CAD build for the part. Positions are in the model's coordinates, mm. A direction names the side the tool comes from. Give positions to 0.01 mm unless a question says otherwise; leave off trailing zeros. Write each loop counter-clockwise with the first axis right and the second up, starting at its lowest first coordinate (ties: lowest second). Pieces come first, ordered by that corner, then holes. Notation, with made-up numbers: (27, 76) - (72, 76) arc R19 ccw to (72, 94) - close; hole circle Ø9 at (-7, 42.25). An arc over 180 degrees is marked (long way). Put each result on its own line as item: value. Start each with the question number.
1. Cut at B-B on x = 0. List the corners of the cut face in (y, z).
2. Mould opens along Y. For faces 1 (the cylindrical face through (-3.88, -17.48, -12.64)), 2 (the flat face through (-4.89, 14, -19)), 3 (the flat face through (-8, -15, -5.426)) say: +Y half, -Y half, draft (parallel to the pull), parting line (faces both ways), or undercut.
3. Drop flat-ended pins along their axis: pin 1 (3 mm diameter, centred on y = 8, z = -9, fed in from +X); pin 2 (8 mm diameter, centred on x = 13.5, z = -18, fed in from -Y); pin 3 (16 mm diameter, centred on x = -5, y = -5.5, fed in from +Z). Give the stop position or say it passes through.
4. Cut at C-C on y = 9.5. List the corners of the cut face in (x, z).
5. Cut at A-A on y = 0. List the corners of the cut face in (x, z), and give its area (3 significant figures).
6. Tool access for faces 4 (the flat face through (4.9, -12.2, -18.126)), 5 (the flat face through (4.89, 14, -19)), 6 (the flat face through (-1.4, -13.2, -19.65)): list every direction of +Z, -Z, +X, -X, +Y, -Y with a clear straight run to the whole face (end or side of a thin tool).
7. Cut at D-D on z = -9.5. List the corners of the cut face in (x, y), and give its area (3 significant figures).
8. Wall check: line 1 (Y direction, x = 0, z = -10.75); line 2 (Z direction, x = -10, y = 12.5); line 3 (X direction, y = -12.5, z = -14). Give the ranges that are in metal, low to high.
from build123d import *

# Parameters (mm, degrees)
CUT_EXTRUDE1_DEPTH = 15.224


with BuildPart() as part:
    # Sketch1 → Revolve1 (revolve)
    with BuildSketch(Plane(origin=(0, 0, 0), x_dir=(1, 0, 0), z_dir=(0, 1, 0))):
        Polygon((16.383, 5.425637802), (17.907, 5.425637802), (17.907, 19.649637802), (12.954, 19.649637802), (12.954, 18.125637802), (16.383, 18.125637802), align=None)
    revolve(axis=Axis((0, 0, -10.179008168), (0, 0, 1)))

    # Sketch2 → Cut-Extrude1 (cut, through all)
    with BuildSketch(Plane(origin=(0, 0, -19.649637802), x_dir=(-1, 0, 0), z_dir=(0, 0, -1))):
        with BuildLine():
            Line((-4.8895, 15.636351197), (-4.8895, 10.556351197))
            Line((-4.8895, 10.556351197), (4.8895, 10.556351197))
            Line((4.8895, 10.556351197), (4.8895, 15.636351197))
            ThreePointArc((4.8895, 15.636351197), (0, 16.383), (-4.8895, 15.636351197))
        make_face()
    extrude(amount=-CUT_EXTRUDE1_DEPTH, mode=Mode.SUBTRACT)


solid = part.part
Report:
1. outline: (-17.91, -19.65) - (-12.95, -19.65) - (-12.95, -18.13) - (-16.38, -18.13) - (-16.38, -5.43) - (-17.91, -5.43) - close; (16.38, -19.65) - (17.91, -19.65) - (17.91, -5.43) - (16.38, -5.43) - close
2. face 1: parting line
2. face 2: undercut
2. face 3: draft
3. pin 1: stops at x = 16.69
3. pin 2: stops at y = -15.18
3. pin 3: stops at z = -18.13
4. outline: (-15.18, -19.65) - (-8.81, -19.65) - (-8.81, -18.13) - (-13.35, -18.13) - (-13.35, -5.43) - (-15.18, -5.43) - close; (8.81, -19.65) - (15.18, -19.65) - (15.18, -5.43) - (13.35, -5.43) - (13.35, -18.13) - (8.81, -18.13) - close
5. outline: (-17.91, -19.65) - (-12.95, -19.65) - (-12.95, -18.13) - (-16.38, -18.13) - (-16.38, -5.43) - (-17.91, -5.43) - close; (12.95, -19.65) - (17.91, -19.65) - (17.91, -5.43) - (16.38, -5.43) - (16.38, -18.13) - (12.95, -18.13) - close
5. area: 53.8 mm²
6. face 4: +Z
6. face 5: +Z, -Z
6. face 6: -Z, +X, -X, +Y, -Y
7. outline: circle Ø35.81 at (0, 0); hole circle Ø32.77 at (0, 0)
7. area: 164 mm²
8. line 1: y = -17.91 to -16.38, 16.38 to 17.91
8. line 2: z = -19.65 to -18.13
8. line 3: x = -12.82 to -10.59, 10.59 to 12.82
